Source: three-view drawing plus pictorial views. Frame: mm from the lowest corner of the part. A direction names the side the tool comes from. Round coordinates to 2 decimals unless told otherwise and drop trailing zeros. Order: outer loops, then holes, each group sorted by start corner. A loop starts at its lowest first (then second) coordinate and runs counter-clockwise, first axis right, second up. Notation, with made-up numbers: (50, -19.75) -> (108, -19.75) arc R23 ccw to (108, -0.75) -> close; hole circle Ø3 at (56, 35.5). An arc over 180 degrees is marked (long way). Answer as CSV lines item,"result".
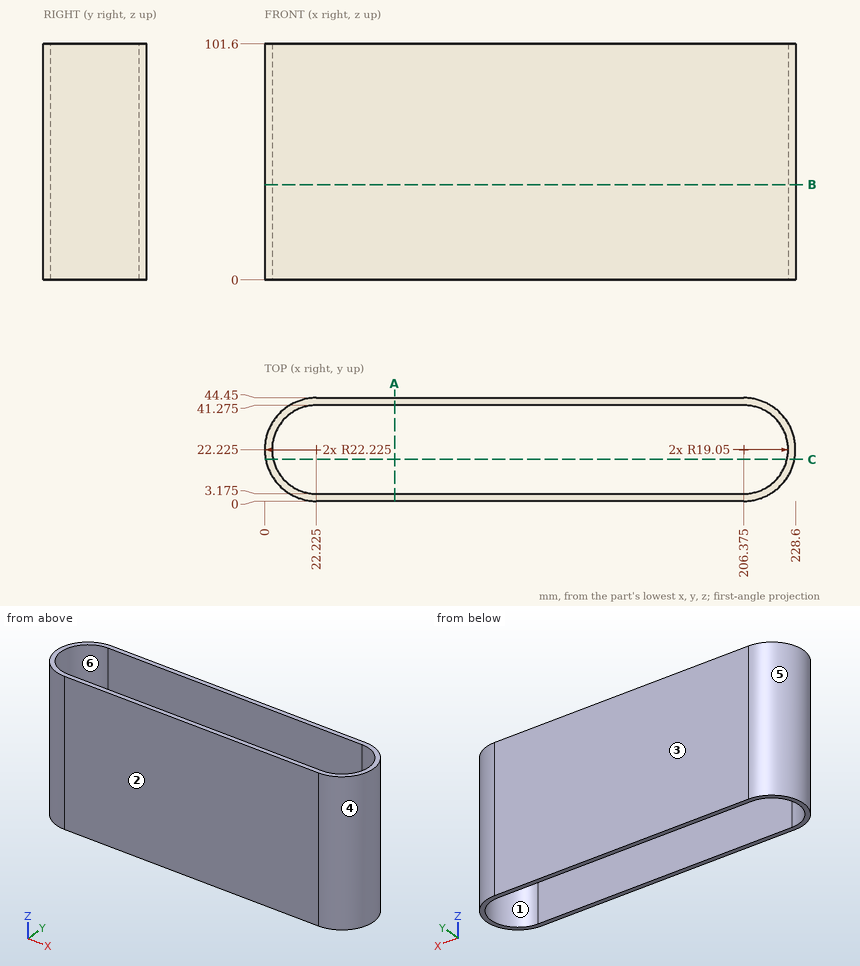
1. Line query: L1, parallel to Y at x = 37, z = 79 (3 decimals); L2, parallel to X at y = 22.5, z = 25; L3, parallel to X at y = 29.5, z = 52. Output: solid intervals per line, ascending. Write a range as [from, to].
Results below:
L1,"[0, 3.175], [41.275, 44.45]"
L2,"[0, 3.18], [225.42, 228.6]"
L3,"[1.22, 4.62], [223.98, 227.38]"
2. Reachability of the marked faces 5 and 6 from +Z, -Z, +X, -X, +Y, -Y: full face, straight path, thin tool, end or side. Return the list, or none.
Results below:
face 5,"+Z, -Z, -X"
face 6,"+Z, -Z"
3. Pin query (flat end, axial travel): pin 1 (5 mm diameter, centred on y = 17.5, z = 44.5, fed in from +X); pin 2 (8 mm diameter, centred on y = 39.5, z = 49, fed in from -X); pin 3 (12 mm diameter, centred on y = 24, z = 31, fed in from -X); pin 4 (2 mm diameter, centred on x = 43.5, y = 38.5, fed in from +Z). Return the tip coordinate at first contact, or that it passes through.
Results below:
pin 1,"x = 228.49"
pin 2,"x = 4.4"
pin 3,"x = 0"
pin 4,"through"
4. Mould query, pull axis Y, two halves, no side actions, for the marked faces 1, 2, 3 and 4. Classes: released by +Y, released by -Y, zero draft, split by the parting line, or undercut.
Results below:
face 1,"undercut"
face 2,"released by -Y"
face 3,"released by +Y"
face 4,"split by the parting line"
5. Section query B-B on z = 41. Return loops of the section in (x, y) (3 decimals), and give its area (3 significant figures).
Results below:
outline,"(22.225, 0) -> (206.375, 0) arc R22.225 ccw to (206.375, 44.45) -> (22.225, 44.45) arc R22.225 ccw to start; hole (22.225, 3.175) -> (206.375, 3.175) arc R19.05 ccw to (206.375, 41.275) -> (22.225, 41.275) arc R19.05 ccw to start"
area,"1,580 mm2"
6. Section query A-A on x = 56. Return loops of the section in (y, z) (3 decimals), and give its area (3 significant figures).
Results below:
outline,"(0, 0) -> (3.175, 0) -> (3.175, 101.6) -> (0, 101.6) -> close; (41.275, 0) -> (44.45, 0) -> (44.45, 101.6) -> (41.275, 101.6) -> close"
area,"645 mm2"
7. Section query C-C on y = 18. Return loops of the section in (x, z).
Results below:
outline,"(0.41, 0) -> (3.65, 0) -> (3.65, 101.6) -> (0.41, 101.6) -> close; (224.95, 0) -> (228.19, 0) -> (228.19, 101.6) -> (224.95, 101.6) -> close"
